The listing builds one solid part. Answer for the finished solid, in the listing's coordinates (mm). A direction names the side the tool comes from. Coordinates: 2 decimals unless noted, no trailing zeros. Loops run counter-clockwise (first coordinate to the right, second up) from the corner with the lowest first, then second, coordinate; pieces in that order, holes last. Notation, with made-up numbers: (-38.5, -2.75) -> (18.5, -2.75) arc R19 ccw to (18.5, 24.25) -> close; hole circle Ø2 at (-40, -22). An arc over 180 degrees is marked (long way). Answer in a Markdown table with one row per item.
Autodesk Inventor part; units mm, degrees
ref_plane "YZ Plane" through (0, 0, 0) normal (1, 0, 0) x (0, 1, 0)
ref_plane "XZ Plane" through (0, 0, 0) normal (0, 1, 0) x (-1, 0, 0)
ref_plane "XY Plane" through (0, 0, 0) normal (0, 0, 1) x (1, 0, 0)
sketch "Sketch1" plane through (0, 0, 0) normal (0, 0, 1) x (1, 0, 0)
  line L0 (-6.35, -3.6662) -> (-6.35, 3.6662)
  line L1 (-6.35, 3.6662) -> (0, 7.3323)
  line L2 (0, 7.3323) -> (6.35, 3.6662)
  line L3 (6.35, 3.6662) -> (6.35, -3.6662)
  line L4 (6.35, -3.6662) -> (0, -7.3323)
  line L5 (0, -7.3323) -> (-6.35, -3.6662)
  point P0 (0, 0)
  point P1 (0, 0)
  dimension "Size" = 12.7
extrude "Extrusion1" add sketch "Sketch1" along normal mid plane 79.375
sketch "Sketch3" plane through (0, 0, 39.6875) normal (0, 0, 1) x (1, 0, 0)
  line L0 (-6.35, 3.6662) -> (0, 7.3323) construction
  line L1 (0, 7.3323) -> (6.35, 3.6662) construction
  line L2 (6.35, 3.6662) -> (6.35, -3.6662) construction
  line L3 (6.35, -3.6662) -> (0, -7.3323) construction
  line L4 (0, -7.3323) -> (-6.35, -3.6662) construction
  line L5 (-6.35, -3.6662) -> (-6.35, 3.6662) construction
  point P0 (0, 0)
hole "Hole1" at (0, 0, 39.6875) direction (0, 0, -1) diameter 5.1054 end through all
sketch "Sketch4" plane through (0, 0, 39.6875) normal (0, 0, 1) x (1, 0, 0)
  circle A0 centre (0, 0) radius 2.5527 construction
  line L0 (-6.35, 3.6662) -> (0, 7.3323) construction
  line L1 (0, 7.3323) -> (6.35, 3.6662) construction
  line L2 (6.35, 3.6662) -> (6.35, -3.6662) construction
  line L3 (6.35, -3.6662) -> (0, -7.3323) construction
  line L4 (0, -7.3323) -> (-6.35, -3.6662) construction
  line L5 (-6.35, -3.6662) -> (-6.35, 3.6662) construction
  circle A1 centre (0, 0) radius 6.8771
  circle A2 centre (0, 0) radius 8.89
  dimension "thunder" = 13.7541
  dimension "d16" = 17.78
extrude "Extrusion3" cut sketch "Sketch4" against normal through all
sketch "Sketch5" plane through (0, 0, 39.6875) normal (0, 0, 1) x (1, 0, 0)
  arc A0 (5.4616, -4.1791) -> (6.35, -2.6403) centre (0, 0) ccw
  line L0 (5.4616, -4.1791) -> (0.8884, -6.8194)
  arc A1 (-0.8884, -6.8194) -> (0.8884, -6.8194) centre (0, 0) ccw
  line L1 (-0.8884, -6.8194) -> (-5.4616, -4.1791)
  arc A2 (-6.35, -2.6403) -> (-5.4616, -4.1791) centre (0, 0) ccw
  line L2 (-6.35, -2.6403) -> (-6.35, 2.6403)
  arc A3 (-5.4616, 4.1791) -> (-6.35, 2.6403) centre (0, 0) ccw
  line L3 (-5.4616, 4.1791) -> (-0.8884, 6.8194)
  arc A4 (0.8884, 6.8194) -> (-0.8884, 6.8194) centre (0, 0) ccw
  line L4 (0.8884, 6.8194) -> (5.4616, 4.1791)
  arc A5 (6.35, 2.6403) -> (5.4616, 4.1791) centre (0, 0) ccw
  line L5 (6.35, 2.6403) -> (6.35, -2.6403)
  circle A6 centre (0, 0) radius 2.5527
  circle A7 centre (0, 0) radius 6.35
  point P0 (-3.175, 5.4993)
  point P1 (3.175, 5.4993)
  point P2 (6.35, 0)
  point P3 (-6.35, 0)
  point P4 (-3.175, -5.4993)
  point P5 (3.175, -5.4993)
  dimension "d19" = 12.7
extrude "Extrusion4" cut sketch "Sketch5" against normal blind 8.001 contours L0 A7 L5 A0 | L0 A1 L1 A7 | A7 L4 A5 L5 | L1 A2 L2 A7 | A7 L3 A4 L4 | L2 A3 L3 A7
mirror "Mirror2" about plane through (0, 0, 0) normal (0, 0, 1) of "Extrusion4"
equation "\"bearing\" = 25.4"
properties part number "CL4-011" material "Aluminum 6061"
Item 1: Find the intervals of material crossed by probe 1 along X at (y, z) = (0, -9.5); probe 2 along Y at (x, z) = (0, 11.5); probe 3 along Y at (x, z) = (0.25, -3), in increasing order.
Findings below:
| item | result |
|---|---|
| probe 1 | x = -6.35 to -2.55, 2.55 to 6.35 |
| probe 2 | y = -6.88 to -2.55, 2.55 to 6.88 |
| probe 3 | y = -6.87 to -2.54, 2.54 to 6.87 |
Item 2: A cutting plane is placed at B-B, the plane z = 30.5. Determine the outline of the cut face in (x, y), plus the area to 3 significant figures.
Findings below:
| item | result |
|---|---|
| outline | (-6.35, -2.64) arc R6.88 ccw to (-5.46, -4.18) -> (-0.89, -6.82) arc R6.88 ccw to (0.89, -6.82) -> (5.46, -4.18) arc R6.88 ccw to (6.35, -2.64) -> (6.35, 2.64) arc R6.88 ccw to (5.46, 4.18) -> (0.89, 6.82) arc R6.88 ccw to (-0.89, 6.82) -> (-5.46, 4.18) arc R6.88 ccw to (-6.35, 2.64) -> close; hole circle Ø5.11 at (0, 0) |
| area | 117 mm2 |
Item 3: Determine the mould class of faces 1 (the face through (-3.21, 5.48, -0.44)), 2 (the face through (3.21, -5.48, -0.44)), 3 (the face through (-6.35, 0, 0)), 4 (the face through (-0.767, -2.435, -0.556)) for opening direction Y: +Y half, -Y half, draft (parallel to the pull), parting line (faces both ways), or undercut.
Findings below:
| item | result |
|---|---|
| face 1 | +Y half |
| face 2 | -Y half |
| face 3 | draft |
| face 4 | undercut |
Item 4: Flat-ended cylindrical pins translate along their axes: pin 1 Ø1.5 at (y, z) = (-4, -15.5) entering from +X; pin 2 Ø3.5 at (x, y) = (-5.5, -4) entering from +Z; pin 3 Ø2 at (x, z) = (-4.5, -25) entering from -Y. Find the tip coordinate at first contact, or state that the pin passes through.
Findings below:
| item | result |
|---|---|
| pin 1 | stops at x = 6.06 |
| pin 2 | stops at z = 39.69 |
| pin 3 | stops at y = -5.31 |
Item 5: A cutting plane is placed at A-A, the plane x = 1.75. Determine the outline of the cut face in (y, z).
Findings below:
| item | result |
|---|---|
| outline | (-6.32, -31.69) -> (-6.1, -31.69) -> (-6.1, -39.69) -> (-1.86, -39.69) -> (-1.86, 39.69) -> (-6.1, 39.69) -> (-6.1, 31.69) -> (-6.32, 31.69) -> close; (1.86, -39.69) -> (6.1, -39.69) -> (6.1, -31.69) -> (6.32, -31.69) -> (6.32, 31.69) -> (6.1, 31.69) -> (6.1, 39.69) -> (1.86, 39.69) -> close |
Item 6: A tool of negligible diameter and unlimited length cuts with its end or side. For faces 5 (the face through (6, 3, -31.686)), 6 (the face through (0, 6.5, 31.686)), 7 (the face through (-6, -3, 31.686)), 8 (the face through (-1.38, 6.2, -35.74)), 9 (the face through (6, -3, 31.686)), from which of +Z, -Z, +X, -X, +Y, -Y can it reach the whole face along a straight path? Write none if from no direction.
Findings below:
| item | result |
|---|---|
| face 5 | -Z, +X, +Y |
| face 6 | +Z, +Y |
| face 7 | +Z, -X, -Y |
| face 8 | -Z |
| face 9 | +Z, +X, -Y |
